from build123d import *

# Parameters (mm, degrees)
SKETCH1_W           = 11.5
SKETCH1_H           = 11.5
BOSS_EXTRUDE1_DEPTH = 338.5
SKETCH2_W           = 11.5
SKETCH2_H           = 11.5
BOSS_EXTRUDE2_DEPTH = 100
FILLET1_R           = 40
FILLET2_R           = 51.5
FILLET3_R           = 6


with BuildPart() as part:
    # Sketch1 → Boss-Extrude1 (new body)
    with BuildSketch(Plane.XY):
        Rectangle(SKETCH1_W, SKETCH1_H)
    extrude(amount=BOSS_EXTRUDE1_DEPTH)

    # Sketch2 → Boss-Extrude2 (add)
    with BuildSketch(Plane.ZY.offset(5.75)):
        with Locations((5.75, 0)):
            Rectangle(SKETCH2_W, SKETCH2_H)
    extrude(amount=BOSS_EXTRUDE2_DEPTH)

    # Fillet1
    fillet1_edges = [part.edges().sort_by_distance(p)[0] for p in [
        (-5.75, 0, 11.5),
    ]]
    fillet(fillet1_edges, radius=FILLET1_R)

    # Fillet2
    fillet2_edges = [part.edges().sort_by_distance(p)[0] for p in [
        (5.75, 0, 0),
    ]]
    fillet(fillet2_edges, radius=FILLET2_R)

    # Fillet3
    # the kernel refuses this fillet: 6 mm, written as the material it takes off along each edge
    with BuildSketch(Plane(origin=(-5.75, -5.75, 51.5), x_dir=(0, 1, 0), z_dir=(0, 0, 1)), Plane(origin=(-5.75, 5.75, 51.5), x_dir=(1, 0, 0), z_dir=(0, 0, 1))) as fillet3_piece_1:
        with BuildLine():
            CenterArc((FILLET3_R, -FILLET3_R), FILLET3_R, 90, 90)
            Line((0, -FILLET3_R), (0, 0))
            Line((0, 0), (FILLET3_R, 0))
        make_face()
    extrude(amount=302, mode=Mode.SUBTRACT)
    with BuildSketch(Plane(origin=(-45.75, -5.75, 51.5), x_dir=(0, 0, -1), z_dir=(-1, 0, 0))) as fillet3_piece_2:
        with BuildLine():
            CenterArc((40 + FILLET3_R, -FILLET3_R), FILLET3_R, 90, 90)
            Line((40 + FILLET3_R, 0), (40, 0))
            Line((40, 0), (40, -FILLET3_R))
        make_face()
    revolve(axis=Axis((-45.75, -5.75, 51.5), (0, -1, 0)), revolution_arc=90, mode=Mode.SUBTRACT)
    with BuildSketch(Plane(origin=(-45.75, 5.75, 51.5), x_dir=(0, 0, -1), z_dir=(-1, 0, 0))) as fillet3_piece_3:
        with BuildLine():
            CenterArc((40 + FILLET3_R, FILLET3_R), FILLET3_R, 180, 90)
            Line((40, FILLET3_R), (40, 0))
            Line((40, 0), (40 + FILLET3_R, 0))
        make_face()
    revolve(axis=Axis((-45.75, 5.75, 51.5), (0, -1, 0)), revolution_arc=90, mode=Mode.SUBTRACT)
    with BuildSketch(Plane(origin=(5.75, -5.75, 51.5), x_dir=(0, 1, 0), z_dir=(0, 0, 1)), Plane(origin=(5.75, 5.75, 51.5), x_dir=(-1, 0, 0), z_dir=(0, 0, 1))) as fillet3_piece_4:
        with BuildLine():
            CenterArc((FILLET3_R, FILLET3_R), FILLET3_R, 180, 90)
            Line((0, FILLET3_R), (0, 0))
            Line((0, 0), (FILLET3_R, 0))
        make_face()
    extrude(amount=302, mode=Mode.SUBTRACT)
    with BuildSketch(Plane(origin=(-45.75, -5.75, 51.5), x_dir=(1, 0, 0), z_dir=(0, 0, 1))) as fillet3_piece_5:
        with BuildLine():
            CenterArc((51.5 - FILLET3_R, FILLET3_R), FILLET3_R, 270, 90)
            Line((51.5 - FILLET3_R, 0), (51.5, 0))
            Line((51.5, 0), (51.5, FILLET3_R))
        make_face()
    revolve(axis=Axis((-45.75, -5.75, 51.5), (0, 1, 0)), revolution_arc=90, mode=Mode.SUBTRACT)
    with BuildSketch(Plane(origin=(-45.75, 5.75, 51.5), x_dir=(1, 0, 0), z_dir=(0, 0, 1))) as fillet3_piece_6:
        with BuildLine():
            CenterArc((51.5 - FILLET3_R, -FILLET3_R), FILLET3_R, 0, 90)
            Line((51.5, -FILLET3_R), (51.5, 0))
            Line((51.5, 0), (51.5 - FILLET3_R, 0))
        make_face()
    revolve(axis=Axis((-45.75, 5.75, 51.5), (0, 1, 0)), revolution_arc=90, mode=Mode.SUBTRACT)
    with BuildSketch(Plane(origin=(-45.75, -5.75, 11.5), x_dir=(0, 1, 0), z_dir=(-1, 0, 0)), Plane(origin=(-45.75, 5.75, 11.5), x_dir=(0, 0, -1), z_dir=(-1, 0, 0))) as fillet3_piece_7:
        with BuildLine():
            CenterArc((FILLET3_R, FILLET3_R), FILLET3_R, 180, 90)
            Line((0, FILLET3_R), (0, 0))
            Line((0, 0), (FILLET3_R, 0))
        make_face()
    extrude(amount=75, mode=Mode.SUBTRACT)
    with BuildSketch(Plane(origin=(-45.75, -5.75, 0), x_dir=(0, 1, 0), z_dir=(-1, 0, 0)), Plane(origin=(-45.75, 5.75, 0), x_dir=(0, 0, 1), z_dir=(-1, 0, 0))) as fillet3_piece_8:
        with BuildLine():
            CenterArc((FILLET3_R, -FILLET3_R), FILLET3_R, 90, 90)
            Line((0, -FILLET3_R), (0, 0))
            Line((0, 0), (FILLET3_R, 0))
        make_face()
    extrude(amount=75, mode=Mode.SUBTRACT)


solid = part.part
Geometry: final body of the model. Coordinates: model frame, mm. A direction names the side the tool comes from. Round coordinates to 2 decimals unless told otherwise and drop trailing zeros. Loops run counter-clockwise (first coordinate to the right, second up) from the corner with the lowest first, then second, coordinate; pieces in that order, holes last. Notation, with made-up numbers: M 80,38.5 L 109,38.5 A20 cw 109,69.5 Z; hole C 89.5,63.5 d9. An arc over 180 degrees is marked long. Put each result on its own line as item: value. Start each with the question number.
(1) Section query C-C (z = 227). Return loops of the section in (x, y).
(2) Set-up query: faces 1 (the face through (0, 0, 338.5)), 2 (the face through (-75.33, -4.037, 9.698)), 3 (the face through (-75.33, 3.948, 9.787)). Return all of +Z, -Z, +X, -X, +Y, -Y with unobstructed straight access to the full face (end or side cutting, diameter ignored); none if empty.
(3) Material intervals for line 1 along Z through (x, y) = (-70, -0.5); line 2 along X through (y, z) = (2, 252); line 3 along Z through (x, y) = (-61, 4.5), sorted ascending. Write a range as [from, to].
(4) Section query B-B (x = -75.5). Return loops of the section in (y, z).
(5) Section query A-A (y = -2). Return loops of the section in (x, z), then the cut area to 3 significant figures.
(6) Contact query for flat-ended pins moving along their axis: pin 1 Ø3 at (y, z) = (-4.5, 264) entering from +X; pin 2 Ø2 at (y, z) = (-2.5, 165) entering from -X; pin 3 Ø4 at (x, y) = (-16, 4) entering from +Z; pin 4 Ø10 at (x, z) = (-14.5, 273) entering from +Y. Output: stop coordinate, or through.
Findings below:
1. outline: M -5.74,0 A6 ccw 0,-5.74 A6 ccw 5.74,0 A6 ccw 0,5.74 A6 ccw Z
2. face 1: +Z, +X, -X, +Y, -Y
2. face 2: +Z, -X, -Y
2. face 3: +Z, -X, +Y
3. line 1: z = [0.05, 11.45]
3. line 2: x = [-5.31, 5.31]
3. line 3: z = [2.33, 9.17]
4. outline: M -5.74,5.75 A6 ccw 0,0.01 A6 ccw 5.74,5.75 A6 ccw 0,11.49 A6 ccw Z
5. outline: M -105.75,0.44 L -45.75,0.44 A51.06 ccw 5.31,51.5 L 5.31,338.5 L -5.31,338.5 L -5.31,51.5 A40.44 cw -45.75,11.06 L -105.75,11.06 Z
5. area: 4,450 mm2
6. pin 1: stops at x = 4.79
6. pin 2: stops at x = -5.49
6. pin 3: stops at z = 25.34
6. pin 4: passes through
